```python
from build123d import *

# Parameters (mm, degrees)
CYLINDER_R             = 4
CYLINDER_DEPTH         = 125
BOX003_W               = 8
BOX003_H               = 125
BOX003_DEPTH           = 2
BOX002_W               = 90
BOX002_H               = 125
BOX002_DEPTH           = 50
BOX002_PLACEMENT_ANGLE = 10
BOX001_W               = 85
BOX001_H               = 105
BOX001_DEPTH           = 13
BOX001_PLACEMENT_ANGLE = 356
BOX_W                  = 80
BOX_H                  = 125
BOX_DEPTH              = 50


with BuildPart() as mount_hole:
    # Cylinder → Cylinder (new body)
    with BuildSketch(Plane(origin=(60, 0, 6), x_dir=(1, 0, 0), z_dir=(0, 1, 0))):
        Circle(CYLINDER_R)
    extrude(amount=CYLINDER_DEPTH)


with BuildPart() as edge_remove:
    # Box003 → Box003 (new body)
    with BuildSketch(Plane.XY):
        with Locations((4, 62.5)):
            Rectangle(BOX003_W, BOX003_H)
    extrude(amount=BOX003_DEPTH)


with BuildPart() as guide_cutout:
    # Box002 → Box002 (new body)
    with BuildSketch(Plane.XY):
        with Locations((45, 62.5)):
            Rectangle(BOX002_W, BOX002_H)
    extrude(amount=BOX002_DEPTH)


with BuildPart() as guide_cutout_1:
    # Box002 placement: moved
    add(guide_cutout.part.rotate(Axis((0, 0, 0), (0, -1, 0)), BOX002_PLACEMENT_ANGLE))


with BuildPart() as belt_cutout:
    # Box001 → Box001 (new body)
    with BuildSketch(Plane.XY):
        with Locations((42.5, 52.5)):
            Rectangle(BOX001_W, BOX001_H)
    extrude(amount=BOX001_DEPTH)


with BuildPart() as belt_cutout_1:
    # Box001 placement: moved
    add(belt_cutout.part.moved(Location((0, 10, -13))).rotate(Axis((0, 10, -13), (0, 1, 0)), BOX001_PLACEMENT_ANGLE))


with BuildPart() as cut003:
    # Box → Box (new body)
    with BuildSketch(Plane.XY):
        with Locations((40, 62.5)):
            Rectangle(BOX_W, BOX_H)
    extrude(amount=BOX_DEPTH)

    # Cut: cut belt_cutout
    add(belt_cutout_1.part, mode=Mode.SUBTRACT)

    # Cut001: cut guide_cutout
    add(guide_cutout_1.part, mode=Mode.SUBTRACT)

    # Cut002: cut edge_remove
    add(edge_remove.part, mode=Mode.SUBTRACT)

    # Cut003: cut mount_hole
    add(mount_hole.part, mode=Mode.SUBTRACT)


solid = cut003.part
```
For this review, take the finished solid that the model builds, in its own axes (mm). A direction names the side the tool comes from. Coordinates: 2 decimals unless noted, no trailing zeros. Write each loop counter-clockwise with the first axis right and the second up, starting at its lowest first coordinate (ties: lowest second). Pieces come first, ordered by that corner, then holes. Notation, with made-up numbers: (10, 38) -> (18, 38) arc R21 ccw to (18, 61) -> close; hole circle Ø9 at (2.5, -11.75). An arc over 180 degrees is marked (long way). Put each result on its own line as item: value.
Q1. Take a section at A-A, the plane z = 8.5. State the section outline as (x, y) points.
From the geometry:
outline: (48.21, 0) -> (56.88, 0) -> (56.88, 125) -> (48.21, 125) -> close; (63.12, 0) -> (80, 0) -> (80, 125) -> (63.12, 125) -> close
Q2. The part is to be moulded in two halves that separate along Y. For faces 3 (the flat face through (31.932, 63.235, 2.265)), 4 (the flat face through (51, 125, 5)), 5 (the flat face through (80, 62, 9)), say which applies: +Y half, -Y half, draft (parallel to the pull), parting line (faces both ways), or undercut.
From the geometry:
face 3: undercut
face 4: +Y half
face 5: draft
Q3. Tool access review of faces 1 (the flat face through (51, 0, 5)), 2 (the flat face through (71.74, 63.24, 5.05)): name each direction out of +Z, -Z, +X, -X, +Y, -Y from which nothing blocks a thin tool from reaching the whole face with its end or side.
From the geometry:
face 1: +Z, -Z, +X, -X, -Y
face 2: -Z, +X
Q4. Take a section at B-B, the plane x = 60. State the section outline as (y, z) points.
From the geometry:
outline: (0, 0) -> (10, 0) -> (10, 2) -> (0, 2) -> close; (0, 10) -> (125, 10) -> (125, 10.58) -> (0, 10.58) -> close; (115, 0) -> (125, 0) -> (125, 2) -> (115, 2) -> close
Q5. Take a section at D-D, the plane x = 38. State the section outline as (y, z) points.
From the geometry:
outline: (0, 0) -> (10, 0) -> (10, 2.69) -> (115, 2.69) -> (115, 0) -> (125, 0) -> (125, 6.7) -> (0, 6.7) -> close
Q6. Clearance check with flat-ended pins moving along their axes: pin 1 Ø3 at (x, y) = (30, 56.5) entering from -Z; pin 2 Ø12 at (x, y) = (64, 19.5) entering from +Z; pin 3 Ø1.5 at (x, y) = (21, 42.5) entering from +Z. State where each tip first meets the part, or that it passes through.
From the geometry:
pin 1: stops at z = 2.02
pin 2: stops at z = 12.34
pin 3: stops at z = 3.84
Q7. Take a section at C-C, the plane y = 50.5. State the section outline as (x, z) points.
From the geometry:
outline: (8, 0.59) -> (56.54, 3.99) arc R4 cw (long way) to (63.7, 4.49) -> (80, 5.63) -> (80, 14.11) -> (8, 1.41) -> close
Q8. Wall thickness on L1, parallel to Y at x = 56, z = 2.5; L2, parallel to Z at x = 34, y = 26; L3, parallel to Z at x = 60, y = 56: over which ranges is each line inside the solid? List them lowest first.
From the geometry:
L1: y = 0 to 10, 115 to 125
L2: z = 2.41 to 6
L3: z = 10 to 10.58
